```python
from build123d import *

# Parameters (mm, degrees)
F0_W        = 87.5617265701
F0_H        = 46.9353795052
F1_DEPTH    = 25.4
F2_R        = 4.9619580549
F3_DEPTH    = 25.4
F4_T1_DEPTH = 72.3353795052
F4_T3_DEPTH = 112.9617265701


# Not quite as in the source:
# - a fillet or chamfer that OpenCascade refuses, or shapes differently, is made with other operations: its cross-section is extruded or revolved along the edge and cut away or added


with BuildPart() as f1:
    # F0 (on Top) → F1 (new body)
    with BuildSketch(Plane.XY):
        with Locations((43.7808632851, 23.4676897526)):
            Rectangle(F0_W, F0_H)
    extrude(amount=F1_DEPTH)

    # F2 (on face) → F3 (cut)
    with BuildSketch(Plane.XY.offset(25.4)):
        with Locations((13.7676307932, 24.1377800703)):
            Circle(F2_R)
    extrude(amount=-F3_DEPTH, mode=Mode.SUBTRACT)

    # F4: fillet of radius 5.08 on 5 edges, made by hand

    # F4_s2 → F4_t1 (cut)
    with BuildSketch(Plane.XZ.offset(-59.6353795052)):
        with BuildLine():
            ThreePointArc((0, 5.08), (1.4878975516, 1.4878975516), (5.08, 0))
            Line((5.08, 0), (0, 0))
            Line((0, 0), (0, 5.08))
        make_face()
        with BuildLine():
            ThreePointArc((82.4817265701, 0), (86.0738290186, 1.4878975516), (87.5617265701, 5.08))
            Line((87.5617265701, 5.08), (87.5617265701, 0))
            Line((87.5617265701, 0), (82.4817265701, 0))
        make_face()
    extrude(amount=F4_T1_DEPTH, mode=Mode.SUBTRACT)

    # F4_s4 → F4_t3 (cut)
    with BuildSketch(Plane.YZ.offset(-12.7)):
        with BuildLine():
            ThreePointArc((46.9353795052, 5.08), (45.4474819536, 1.4878975516), (41.8553795052, 0))
            Line((41.8553795052, 0), (46.9353795052, 0))
            Line((46.9353795052, 0), (46.9353795052, 5.08))
        make_face()
        with BuildLine():
            ThreePointArc((0, 5.08), (1.4878975516, 1.4878975516), (5.08, 0))
            Line((5.08, 0), (0, 0))
            Line((0, 0), (0, 5.08))
        make_face()
    extrude(amount=F4_T3_DEPTH, mode=Mode.SUBTRACT)

    # F4_s5 → F4_t6 (revolve, cut)
    with BuildSketch(Plane.XZ.offset(-24.1377800703)):
        with BuildLine():
            ThreePointArc((23.809588848, 0), (20.2174863996, 1.4878975516), (18.729588848, 5.08))
            Line((18.729588848, 5.08), (18.729588848, 0))
            Line((18.729588848, 0), (23.809588848, 0))
        make_face()
    revolve(axis=Axis((13.7676307932, 24.1377800703, 0), (0, 0, 1)), mode=Mode.SUBTRACT)


solid = f1.part
```
Read the model definition and answer for the solid it produces. Units are mm, in the model's axes. Give positions to 0.01 mm unless a question says otherwise; leave off trailing zeros. Order: outer loops, then holes, each group sorted by start corner. A loop starts at its lowest first (then second) coordinate and runs counter-clockwise, first axis right, second up. Notation, with made-up numbers: (81.25, 11) -> (134.25, 11) arc R8 ccw to (134.25, 26) -> close; hole circle Ø9 at (30, 25.5). An arc over 180 degrees is marked (long way). Write item = value, one per line.
1. A cutting plane is placed at B-B, the plane z = 3. Write down the section's boundary in (x, y).
Numbers:
outline = (0.45, 0.45) -> (87.12, 0.45) -> (87.12, 46.49) -> (0.45, 46.49) -> close; hole circle Ø10.81 at (13.77, 24.14)
2. A cutting plane is placed at A-A, the plane z = 10. Write down the section's boundary in (x, y).
Numbers:
outline = (0, 0) -> (87.56, 0) -> (87.56, 46.94) -> (0, 46.94) -> close; hole circle Ø9.92 at (13.77, 24.14)
3. The mould has two halves that part along X. Classify faces 1 (the face through (0, 23, 15)), 2 (the face through (8.81, 24.36, 15.38)), 3 (the face through (43, 24, 25.4)): +X half, -X half, draft (parallel to the pull), parting line (faces both ways), or undercut.
Numbers:
face_1 = -X half
face_2 = undercut
face_3 = draft
4. Straight lines are drawn through the part: line 1 along X through (y, z) = (34, 4.75); line 2 along X through (y, z) = (25.5, 19.25); line 3 along Y through (x, z) = (45.5, 1.25). For each, find the intervals that lie inside material, in ascending order.
Numbers:
line_1 = 0.01 to 87.55
line_2 = 0 to 9, 18.54 to 87.56
line_3 = 1.74 to 45.19
